Input: part model. Units: mm. Frame: model coordinates. Give positions to 0.01 mm unless a question says otherwise; leave off trailing zeros. Write each loop counter-clockwise with the first axis right and the second up, starting at its lowest first coordinate (ties: lowest second). Pieces come first, ordered by that corner, then holes. Notation, with made-up numbers: (-6, 16.5) - (5, 16.5) arc R14 cw to (5, 41.5) - close; hole circle Ø3 at (-20.75, 24.5). An arc over 180 degrees is marked (long way). Use a Markdown table: item, result. Add a question column.
1. Section query C-C, the plane y = 3.5. Return loops of the section in (x, z), plus the area to 3 significant figures.
2. Mould query, pull axis Y, two halves, no side actions, for faces 1 (the cylindrical face through (40, 0, 1)), 2 (the flat face through (0, 0, 1)), 3 (the cylindrical face through (3.004, 3.565, 0.764)), 4 (the cylindrical face through (1, -12.2, 0.9)). Classes: released by +Y, released by -Y, zero draft, split by the parting line, or undercut.
3. Section query D-D, the plane y = -0.5. Return loops of the section in (x, z).
4. Material intervals for probe 1 along Y at (x, z) = (3.5, 0.3); probe 2 along X at (y, z) = (3.5, 0.3); probe 3 along Y at (x, z) = (44.5, 1.25), sorted ascending.
5. Pin query (flat end, axial travel): pin 1 (4 mm diameter, centred on x = 11, y = 8, fed in from -Z). Return the tip coordinate at first contact, or that it passes through.
6. Section query B-B, the plane x = 41. Return loops of the section in (y, z).
7. Section query A-A, the plane z = 1.15. Return loops of the section in (x, y), plus the area to 3 significant figures.
Autodesk Inventor part; units mm, degrees
ref_plane "YZ Plane" through (0, 0, 0) normal (1, 0, 0) x (0, 1, 0)
ref_plane "XZ Plane" through (0, 0, 0) normal (0, 1, 0) x (-1, 0, 0)
ref_plane "XY Plane" through (0, 0, 0) normal (0, 0, 1) x (1, 0, 0)
sketch "Эскиз1" plane through (0, 0, 0) normal (0, 0, 1) x (1, 0, 0)
  line L0 (53.25, 13.25) -> (0, 13.25)
  line L1 (0, -13.25) -> (53.25, -13.25)
  arc A0 (53.25, 13.25) -> (53.25, -13.25) centre (53.25, 0) ccw
  line L2 (0, -13.25) -> (0, 13.25)
  line L3 (0, 0) -> (40, 0) construction
  line L4 (0, 0) -> (0, 13.25) construction
  line L5 (0, 13.25) -> (0, 11.25)
  point P0 (20, 0)
  dimension "d0" = 13.25
  dimension "d47" = 40
extrude "Выдавливание3" add sketch "Эскиз1" along normal blind 1.8
fillet "Сопряжение3" radius 0.25 2 edges at (53.25, 13.25, 0.9) (53.25, -13.25, 0.9)
fillet "Сопряжение4" radius 3.5 2 edges at (0, -13.25, 0.9) (0, 13.25, 0.9)
sketch "Эскиз6" plane through (0, 0, 1.8) normal (0, 0, 1) x (1, 0, 0)
  arc A0 (49.6774, 12.7593) -> (49.6774, -12.7593) centre (53.25, 0) ccw construction
  line L0 (40, 0) -> (0, 0) construction
  line L1 (0, -13.25) -> (0, 13.25) construction
  circle A1 centre (3.5, 3.5) radius 0.5
  line L2 (3.5, 3.5) -> (0, 3.5) construction
  line L3 (3.5, 3.5) -> (3.5, 0) construction
  circle A2 centre (3.5, -3.5) radius 0.5
  point P0 (49.6099, -13.25)
  dimension "d58" = 1
  dimension "d59" = 3.5
hole "Отверстие1" at (3.5, -3.5, 1.8) at (3.5, 3.5, 1.8) direction (0, 0, -1) diameter 1 end through all countersink diameter 1.5 countersink angle 90
properties part number "Поршень"
Result sheet:
| question | item | result |
|---|---|---|
| 1 | outline | (0, 0) - (3, 0) - (3, 1.55) - (2.75, 1.8) - (0, 1.8) - close; (4, 0) - (40.47, 0) - (40.47, 1.8) - (4.25, 1.8) - (4, 1.55) - close |
| 1 | area | 71.0 mm² |
| 2 | face 1 | undercut |
| 2 | face 2 | zero draft |
| 2 | face 3 | undercut |
| 2 | face 4 | released by -Y |
| 3 | outline | (0, 0) - (40.01, 0) - (40.01, 1.8) - (0, 1.8) - close |
| 4 | probe 1 | y = -13.25 to -4, -3 to 3, 4 to 13.25 |
| 4 | probe 2 | x = 0 to 3, 4 to 40.47 |
| 4 | probe 3 | y = -13.25 to -9.95, 9.95 to 13.25 |
| 5 | pin 1 | stops at z = 0 |
| 6 | outline | (-13.25, 0) - (-5.05, 0) - (-5.05, 1.8) - (-13.25, 1.8) - close; (5.05, 0) - (13.25, 0) - (13.25, 1.8) - (5.05, 1.8) - close |
| 7 | outline | (0, -9.75) arc R3.5 ccw to (3.5, -13.25) - (49.61, -13.25) arc R0.25 ccw to (49.68, -12.76) arc R13.25 cw to (49.68, 12.76) arc R0.25 ccw to (49.61, 13.25) - (3.5, 13.25) arc R3.5 ccw to (0, 9.75) - close; hole circle Ø1 at (3.5, -3.5); hole circle Ø1 at (3.5, 3.5) |
| 7 | area | 1,130 mm² |
